Check sheet for the modelled part. Datum: model origin and axes. Units: mm. Face numbers are marked on the shaded views. A direction names the side the tool comes from. Round coordinates to 2 decimals unless told otherwise and drop trailing zeros. Loops run counter-clockwise (first coordinate to the right, second up) from the corner with the lowest first, then second, coordinate; pieces in that order, holes last. Notation, with made-up numbers: (70, -0.75) - (87, -0.75) arc R32 ccw to (87, 30.25) - close; hole circle Ø8 at (38.5, 57.25). An arc over 180 degrees is marked (long way). Answer in a Markdown table with one row per item. Add a question column.
(1) Gauge pin test, flat ends, axial feed: pin 1 (2 mm diameter, centred on x = 2.5, z = 2.5, fed in from -Y); pin 2 (0.7 mm diameter, centred on x = 2.5, z = 11, fed in from +Y); pin 3 (1.1 mm diameter, centred on y = 4.5, z = 11.5, fed in from +X). Record the tip position at first contact, or that the pin passes through.
(2) Cross-section at B-B on y = 4. Enter the section's corners in (x, z).
(3) Cross-section at A-A on z = 10.25. Enter the section's corners in (x, y), then the cut area to 3 significant figures.
(4) Thickness scan on line 1 along Z through (x, y) = (2.6, 2.75); line 2 along X through (y, z) = (5, 4.5); line 3 along X through (y, z) = (3.5, 10.25). Record the ranges inside material, lowest first.
(5) Cross-section at C-C on x = 2.5. Enter the section's corners in (y, z).
(6) Access from +Z, -Z, +X, -X, +Y, -Y to the whole of each face (thin tool, end or side, straight path). Record for the marked faces 1, 2 and 3.
(7) Cross-section at D-D on z = 2.5. Enter the section's corners in (x, y).
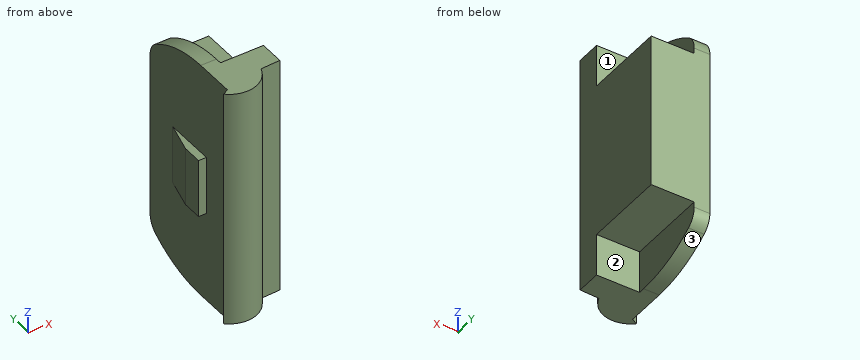
from build123d import *

# Parameters (mm, degrees)
BOSS_EXTRUDE1_DEPTH = 12.3
SKETCH2_W           = 2.2
SKETCH2_H           = 2.17
CUT_EXTRUDE1_DEPTH  = 4.2
CUT_EXTRUDE3_DEPTH  = 0.8
SKETCH5_W           = 3
SKETCH5_H           = 1
BOSS_EXTRUDE2_DEPTH = 0.4
BOSS_EXTRUDE3_DEPTH = 3


with BuildPart() as part:
    # Sketch1 → Boss-Extrude1 (new body)
    with BuildSketch(Plane.XY):
        with BuildLine():
            Line((0, 0), (0.299997713, 0.173208719))
            Line((0.299997713, 0.173208719), (0.299997713, 1.781598719))
            Line((0.299997713, 1.781598719), (0.299997713, 6.107458719))
            Line((0.299997713, 6.107458719), (3.299997713, 6.107458719))
            Line((3.299997713, 6.107458719), (3.299997713, 0.646828719))
            ThreePointArc((3.299997713, 0.646828719), (2.80057856, 0.622710158), (2.301269667, 0.596407591))
            ThreePointArc((2.301269667, 0.596407591), (1.315500673, -0.337939607), (0, 0))
        make_face()
    extrude(amount=BOSS_EXTRUDE1_DEPTH)

    # Sketch2 → Cut-Extrude1 (cut)
    with BuildSketch(Plane(origin=(0, 6.107458719, 0), x_dir=(1, 0, 0), z_dir=(0, 1, 0))):
        with Locations((2.199997713, -1.085)):
            Rectangle(SKETCH2_W, SKETCH2_H)
        with Locations((2.199997713, -11.215)):
            Rectangle(SKETCH2_W, SKETCH2_H)
    extrude(amount=-CUT_EXTRUDE1_DEPTH, mode=Mode.SUBTRACT)

    # Sketch4 → Cut-Extrude3 (cut)
    with BuildSketch(Plane.ZY.offset(-0.299997713)):
        with BuildLine():
            Line((10.41158, 6.107458719), (12.3, 6.107458719))
            Line((12.3, 6.107458719), (12.3, 2.215929667))
            ThreePointArc((12.3, 2.215929667), (12.02880398, 4.022129667), (11.23913234, 5.669043272))
            ThreePointArc((11.23913234, 5.669043272), (10.879869522, 5.991150317), (10.41158, 6.107458719))
        make_face()
        with BuildLine():
            Line((1.88842, 6.107458719), (0, 6.107458719))
            Line((0, 6.107458719), (0, 2.215929667))
            ThreePointArc((0, 2.215929667), (0.27119602, 4.022129667), (1.06086766, 5.669043272))
            ThreePointArc((1.06086766, 5.669043272), (1.420130478, 5.991150317), (1.88842, 6.107458719))
        make_face()
    extrude(amount=-CUT_EXTRUDE3_DEPTH, mode=Mode.SUBTRACT)

    # Sketch5 → Boss-Extrude2 (add)
    with BuildSketch(Plane.ZY.offset(-0.299997713)):
        with Locations((6.15, 2.281598719)):
            Rectangle(SKETCH5_W, SKETCH5_H)
    extrude(amount=BOSS_EXTRUDE2_DEPTH)

    # Sketch6 → Boss-Extrude3 (add)
    with BuildSketch(Plane.XY.offset(7.65)):
        Polygon((0.299997713, 2.781598719), (0.299997713, 4.373208719), (-0.100002287, 2.781598719), align=None)
    extrude(amount=-BOSS_EXTRUDE3_DEPTH)


solid = part.part
Answers:
| question | item | result |
|---|---|---|
| 1 | pin 1 | stops at y = -0.28 |
| 1 | pin 2 | stops at y = 1.91 |
| 1 | pin 3 | stops at x = 1.1 |
| 2 | outline | (0.21, 4.65) - (0.3, 4.65) - (0.3, 0.26) - (1.1, 0.26) - (1.1, 2.17) - (3.3, 2.17) - (3.3, 10.13) - (1.1, 10.13) - (1.1, 12.04) - (0.3, 12.04) - (0.3, 7.65) - (0.21, 7.65) - close |
| 3 | outline | (0, 0) arc R1.4 ccw to (2.3, 0.6) arc R114.32 cw to (3.3, 0.65) - (3.3, 1.91) - (1.1, 1.91) - (1.1, 6.11) - (0.3, 6.11) - (0.3, 0.17) - close |
| 3 | area | 8.90 mm^2 |
| 4 | line 1 | z = 2.17 to 10.13 |
| 4 | line 2 | x = 0.3 to 3.3 |
| 4 | line 3 | x = 0.3 to 1.1 |
| 5 | outline | (0.61, 0) - (1.91, 0) - (1.91, 2.17) - (6.11, 2.17) - (6.11, 10.13) - (1.91, 10.13) - (1.91, 12.3) - (0.61, 12.3) - close |
| 6 | face 1 | +Z, +X, +Y |
| 6 | face 2 | -Z, +X, +Y |
| 6 | face 3 | -Z, +X, -X, +Y |
| 7 | outline | (0, 0) arc R1.4 ccw to (2.3, 0.6) arc R114.32 cw to (3.3, 0.65) - (3.3, 6.11) - (0.3, 6.11) - (0.3, 0.17) - close |
